For this review, use the dimensioned drawing (mm, ordinates from the lowest corner) and the shaded views. A direction names the side the tool comes from. Give positions to 0.01 mm unless a question says otherwise; leave off trailing zeros. Order: outer loops, then holes, each group sorted by start corner. A loop starts at its lowest first (then second) coordinate and runs counter-clockwise, first axis right, second up. Notation, with made-up numbers: (-2.5, 48) -> (49.5, 48) arc R7 cw to (49.5, 59) -> close; hole circle Ø1 at (-3.5, 16.25). An arc over 180 degrees is marked (long way). Answer as a JSON object with one key per item and string values. Group by question number.
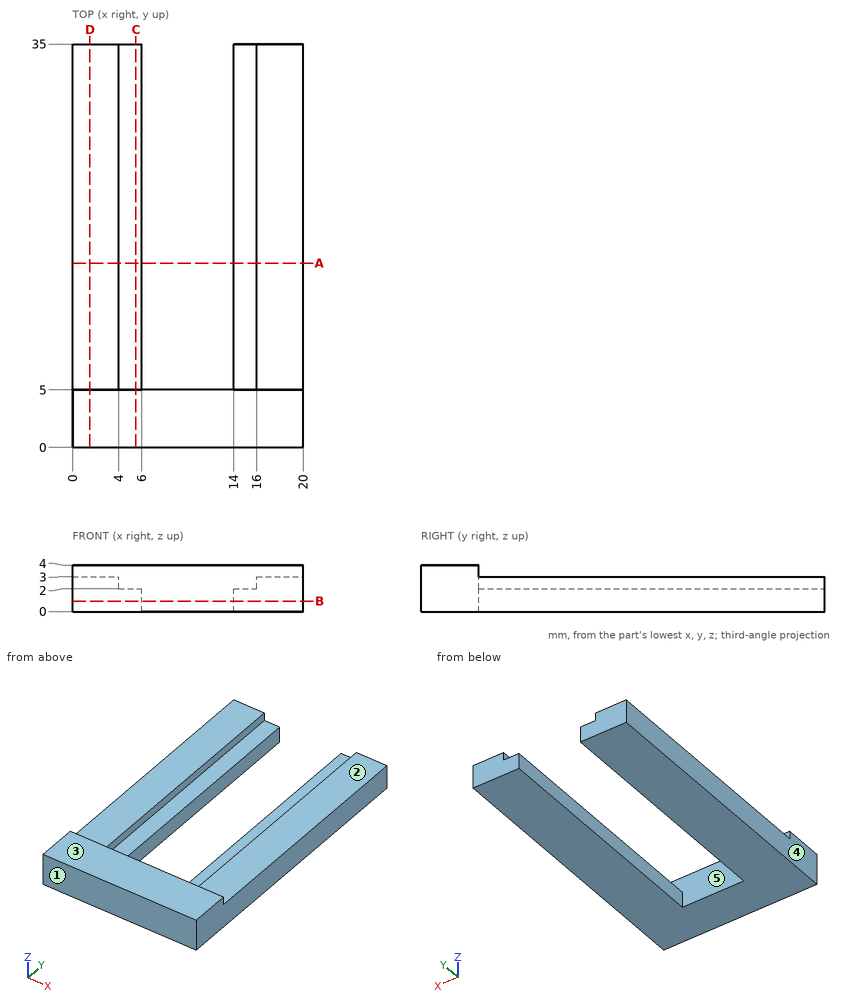
1. Take a section at D-D on x = 1.5. Give the boundary of the cut face in (y, z), plus the area to 3 significant figures.
2. Draft analysis for pull direction X (two halves, no side actions). For the marked faces 3, 4 and 5, state which applies: pulls with the +X half, pulls with the -X half, needs draft (parallel to the pull), parting line crosses it, or undercut.
3. Take a section at C-C on x = 5.5. Give the boundary of the cut face in (y, z), plus the area to 3 significant figures.
4. For probe 1 along X at (y, z) = (12.5, 0.4); probe 2 along X at (y, z) = (20.5, 2.55); probe 3 along Y at (x, z) = (11.75, 0.95), list the stretches that pass through material, from the lowest coordinate up. Write a range as [from, to].
5. Machinability: for the marked faces 1 and 2, which of the approach directions +Z, -Z, +X, -X, +Y, -Y give a long, thin tool a straight path to every point of the face, cutting with its end or side? Answer none if there is none.
6. Take a section at A-A on y = 16. Give the boundary of the cut face in (x, z).
7. For pin 1 (5 mm diameter, centred on x = 10, y = 28.5, fed in from +Z); pin 2 (10 mm diameter, centred on x = 16, y = 24, fed in from +Z), all flat-tipped, find the tip position at first contact; note any pin that passes through.
8. Take a section at B-B on z = 0.9. Give the boundary of the cut face in (x, y), plus the area to 3 significant figures.
Checks:
{
 "1": {"outline": "(0, 0) -> (35, 0) -> (35, 3) -> (5, 3) -> (5, 4) -> (0, 4) -> close", "area": "110 mm2"},
 "2": {"face 3": "needs draft", "face 4": "pulls with the -X half", "face 5": "undercut"},
 "3": {"outline": "(0, 0) -> (35, 0) -> (35, 2) -> (5, 2) -> (5, 4) -> (0, 4) -> close", "area": "80.0 mm2"},
 "4": {"probe 1": "x = [0, 6], [14, 20]", "probe 2": "x = [0, 4], [16, 20]", "probe 3": "y = [0, 5]"},
 "5": {"face 1": "+Z, -Z, +X, -X, -Y", "face 2": "+Z, +X, -X, +Y"},
 "6": {"outline": "(0, 0) -> (6, 0) -> (6, 2) -> (4, 2) -> (4, 3) -> (0, 3) -> close; (14, 0) -> (20, 0) -> (20, 3) -> (16, 3) -> (16, 2) -> (14, 2) -> close"},
 "7": {"pin 1": "passes through", "pin 2": "stops at z = 3"},
 "8": {"outline": "(0, 0) -> (20, 0) -> (20, 35) -> (14, 35) -> (14, 5) -> (6, 5) -> (6, 35) -> (0, 35) -> close", "area": "460 mm2"}
}
